Autodesk Inventor part; units mm, degrees
ref_plane "Work Plane1" through (0, 0, 25.4) normal (0, 0, 1) x (1, 0, 0)
ref_plane "YZ Plane" through (0, 0, 0) normal (1, 0, 0) x (0, 1, 0)
ref_plane "XZ Plane" through (0, 0, 0) normal (0, 1, 0) x (-1, 0, 0)
sketch "Sketch1" plane through (0, 0, 0) normal (0, 1, 0) x (-1, 0, 0)
  line L0 (0, 0) -> (4.388, 0) construction
  line L1 (4.1982, 0) -> (0, 0) construction
  line L2 (0, 0) -> (0, -4.5146) construction
  line L3 (38.1, 38.1) -> (-38.1, 38.1)
  line L4 (-38.1, 38.1) -> (-38.1, -38.1)
  line L5 (-38.1, -38.1) -> (38.1, -38.1)
  line L6 (38.1, -38.1) -> (38.1, 38.1)
  dimension "d0" = 76.2
  dimension "d1" = 76.2
extrude "Extrusion1" add sketch "Sketch1" along normal blind 3.175
ref_plane "Work Plane1" through (0, 0, 25.4) normal (0, 0, 1) x (1, 0, 0)
sketch "Sketch2" plane through (0, 0, 0) normal (0, -1, 0) x (1, 0, 0)
  line L0 (38.1, 38.1) -> (38.1, -38.1)
  line L1 (-38.1, -38.1) -> (-38.1, 38.1)
  line L2 (38.1, 25.3924) -> (-38.1, 25.3924)
  line L3 (-38.1, 25.3924) -> (-38.1, 28.5674)
  line L4 (-38.1, 28.5674) -> (38.1, 28.5674)
  line L5 (38.1, 28.5674) -> (38.1, 25.3924)
  point P0 (0, 0)
  dimension "d5" = 3.175
extrude "Extrusion2" add sketch "Sketch2" along normal blind 25.4
mirror "Mirror1" about plane through (0, 0, 0) normal (0, 0, 1) of "Extrusion2"
sketch "Sketch3" plane through (0, 3.175, 0) normal (0, 1, 0) x (1, 0, 0)
  line L0 (-38.1, 38.1) -> (-38.1, -38.1)
  line L1 (-38.1, -38.1) -> (38.1, -38.1)
  point P0 (0, 0)
  point P1 (-31.75, -31.75)
  dimension "d8" = 6.35
  dimension "d9" = 6.35
hole "Hole1" at (-31.75, 3.175, 31.75) direction (0, -1, 0) diameter 3.175 end through all
mirror "Mirror2" about plane through (0, 0, 0) normal (1, 0, 0) of "Hole1"
mirror "Mirror3" about plane through (0, 0, 0) normal (0, 0, 1) of "Hole1", "Mirror2"
ref_plane "Work Plane2" through (0, 0, 0) normal (0, 0, 1) x (1, 0, 0)
properties part number "Right Angle Frame Mount"
The model under review builds one solid part; all positions refer to its coordinate system, in mm. A direction names the side the tool comes from. Round coordinates to 2 decimals unless told otherwise and drop trailing zeros. Loops run counter-clockwise (first coordinate to the right, second up) from the corner with the lowest first, then second, coordinate; pieces in that order, holes last. Notation, with made-up numbers: (2.5, 79.5) -> (36.5, 79.5) arc R4 ccw to (36.5, 86.5) -> close; hole circle Ø9 at (44.5, -13.75). An arc over 180 degrees is marked (long way). Answer as a JSON object with one key per item and string values. Group by question number.
1) We need section B-B on y = -1. Write out the cut boundary in (x, z), then the cut area to 3 significant figures.
2) We need section A-A on z = -31.75. Write out the cut boundary in (x, y) (1 decimal).
3) For faces 1 (the face through (1, 0, 33)), 2 (the face through (1, -25.4, -27)), 3 (the face through (-1, -13, -25.392)), 4 (the face through (1, -13, -28.567)), list the 3-axis set-ups (+Z, -Z, +X, -X, +Y, -Y) from which the entire face can be reached by the end or side of a thin tool; tool diameter is ignored.
4) For line 1 (X direction, y = 2.4, z = -31.75); line 2 (Z direction, x = -15, y = -17.25), list the stretches that pass through material, from the lowest coordinate up. Write a range as [from, to].
5) For pin 1 Ø12.5 at (x, y) = (18, -9.5) entering from -Z; pin 2 Ø5 at (x, z) = (-2, -32) entering from -Y; pin 3 Ø5 at (x, y) = (11.5, -20.5) entering from +Z; pin 4 Ø5 at (x, z) = (31.75, -31.75) entering from +Y (3 decimals), all flat-tipped, find the tip position at first contact; note any pin that passes through.
6) We need section C-C on x = 17. Write out the cut boundary in (y, z) (3 decimals), then the cut area to 3 significant figures.
7) Mouldability with a two-part tool opening along X and no side actions: class faces 5 (the face through (38.1, 0.5, 5.8)), 6 (the face through (1, 2, -38.1)), 7 (the face through (32.227, 1.565, -33.264)), 8 (the face through (-31.273, 1.565, -33.264)) as released by +X, released by -X, zero draft, split by the parting line, or undercut.
8) We need section D-D on x = 31.75. Write out the cut boundary in (y, z) (1 decimal).
Result set:
{
 "1": {"outline": "(-38.1, -28.57) -> (38.1, -28.57) -> (38.1, -25.39) -> (-38.1, -25.39) -> close; (-38.1, 25.39) -> (38.1, 25.39) -> (38.1, 28.57) -> (-38.1, 28.57) -> close", "area": "484 mm²"},
 "2": {"outline": "(-38.1, 0) -> (-33.3, 0) -> (-33.3, 3.2) -> (-38.1, 3.2) -> close; (-30.2, 0) -> (30.2, 0) -> (30.2, 3.2) -> (-30.2, 3.2) -> close; (33.3, 0) -> (38.1, 0) -> (38.1, 3.2) -> (33.3, 3.2) -> close"},
 "3": {"face 1": "+Z, +X, -X, -Y", "face 2": "+Z, -Z, +X, -X, -Y", "face 3": "+X, -X, -Y", "face 4": "-Z, +X, -X, -Y"},
 "4": {"line 1": "[-38.1, -33.34], [-30.16, 30.16], [33.34, 38.1]", "line 2": "[-28.57, -25.39], [25.39, 28.57]"},
 "5": {"pin 1": "z = -28.57", "pin 2": "y = 0", "pin 3": "z = 28.57", "pin 4": "y = 3.175"},
 "6": {"outline": "(-25.4, -28.567) -> (0, -28.567) -> (0, -38.1) -> (3.175, -38.1) -> (3.175, 38.1) -> (0, 38.1) -> (0, 28.567) -> (-25.4, 28.567) -> (-25.4, 25.392) -> (0, 25.392) -> (0, -25.392) -> (-25.4, -25.392) -> close", "area": "403 mm²"},
 "7": {"face 5": "released by +X", "face 6": "zero draft", "face 7": "undercut", "face 8": "undercut"},
 "8": {"outline": "(-25.4, -28.6) -> (0, -28.6) -> (0, -30.2) -> (3.2, -30.2) -> (3.2, 30.2) -> (0, 30.2) -> (0, 28.6) -> (-25.4, 28.6) -> (-25.4, 25.4) -> (0, 25.4) -> (0, -25.4) -> (-25.4, -25.4) -> close; (0, -38.1) -> (3.2, -38.1) -> (3.2, -33.3) -> (0, -33.3) -> close; (0, 33.3) -> (3.2, 33.3) -> (3.2, 38.1) -> (0, 38.1) -> close"}
}
